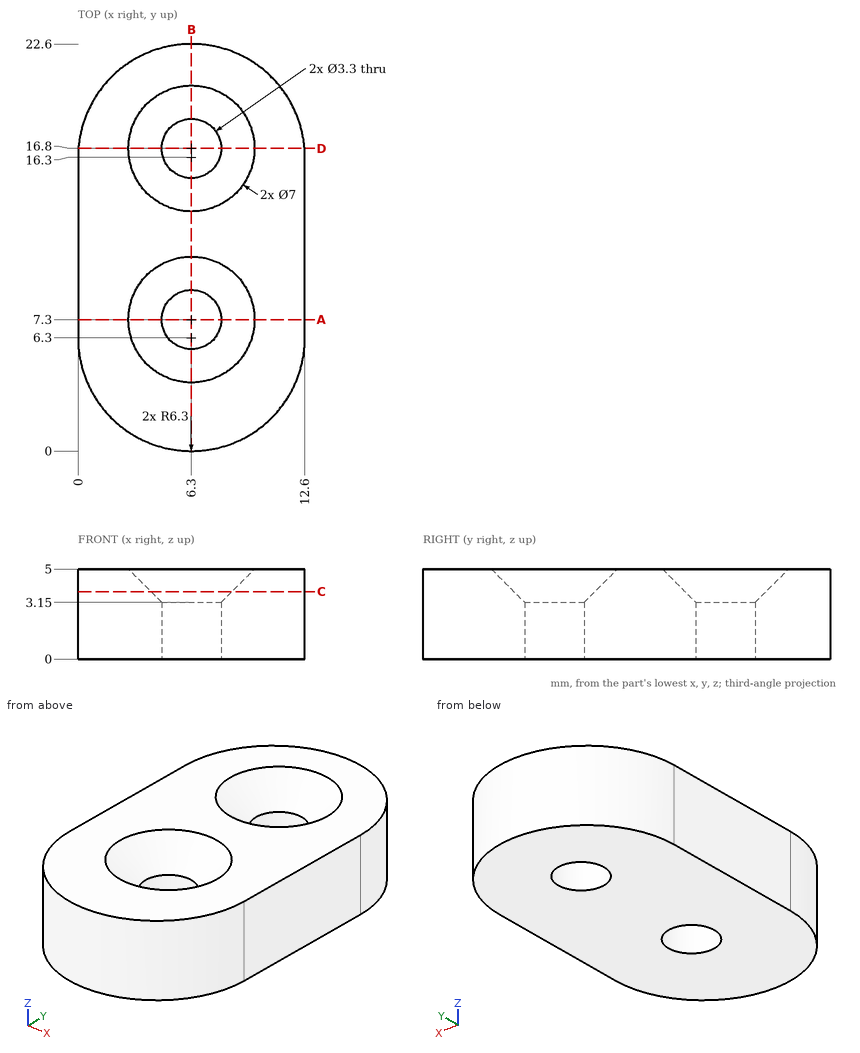
The drawing under review shows one solid part. Ordinate dimensions are in mm from its lowest x, y, z. Round coordinates to 2 decimals unless told otherwise and drop trailing zeros. Loops run counter-clockwise (first coordinate to the right, second up) from the corner with the lowest first, then second, coordinate; pieces in that order, holes last. Notation, with made-up numbers: (10.5, -26) - (50.5, -26) arc R11 ccw to (50.5, -11) - close; hole circle Ø7 at (69.5, 79.25). An arc over 180 degrees is marked (long way). Use one line per item in the form item = value.
Item 1: For line 1 (Y direction, x = 6.3, z = 1); line 2 (Y direction, x = 7.75, z = 2.3); line 3 (X direction, y = 7.3, z = 2.1), list the stretches that pass through material, from the lowest coordinate up.
Answers:
line_1 = 0 to 5.65, 8.95 to 15.15, 18.45 to 22.6
line_2 = 0.17 to 6.51, 8.09 to 16.01, 17.59 to 22.43
line_3 = 0 to 4.65, 7.95 to 12.6
Item 2: Clearance check with flat-ended pins moving along their axes: P1, Ø1, axis at x = 10.5, z = 2.5, coming from the +Y side; P2, Ø1.5, axis at x = 3.5, z = 4, coming from the -Y side. State where each tip first meets the part, or that it passes through.
Answers:
P1 = 21.4
P2 = 0.34
Item 3: Consider section C-C on z = 3.75. Write out the cut boundary in (x, y), then the cut area to 3 significant figures.
Answers:
outline = (0, 6.3) arc R6.3 ccw to (12.6, 6.3) - (12.6, 16.3) arc R6.3 ccw to (0, 16.3) - close; hole circle Ø4.5 at (6.3, 7.3); hole circle Ø4.5 at (6.3, 16.8)
area = 219 mm^2
Item 4: Consider section D-D on y = 16.8. Write out the cut boundary in (x, z), then the cut area to 3 significant figures.
Answers:
outline = (0.02, 0) - (4.65, 0) - (4.65, 3.15) - (2.8, 5) - (0.02, 5) - close; (7.95, 0) - (12.58, 0) - (12.58, 5) - (9.8, 5) - (7.95, 3.15) - close
area = 42.9 mm^2
Item 5: Consider section A-A on y = 7.3. Write out the cut boundary in (x, z).
Answers:
outline = (0, 0) - (4.65, 0) - (4.65, 3.15) - (2.8, 5) - (0, 5) - close; (7.95, 0) - (12.6, 0) - (12.6, 5) - (9.8, 5) - (7.95, 3.15) - close
Item 6: Consider section B-B on x = 6.3. Write out the cut boundary in (y, z).
Answers:
outline = (0, 0) - (5.65, 0) - (5.65, 3.15) - (3.8, 5) - (0, 5) - close; (8.95, 0) - (15.15, 0) - (15.15, 3.15) - (13.3, 5) - (10.8, 5) - (8.95, 3.15) - close; (18.45, 0) - (22.6, 0) - (22.6, 5) - (20.3, 5) - (18.45, 3.15) - close
